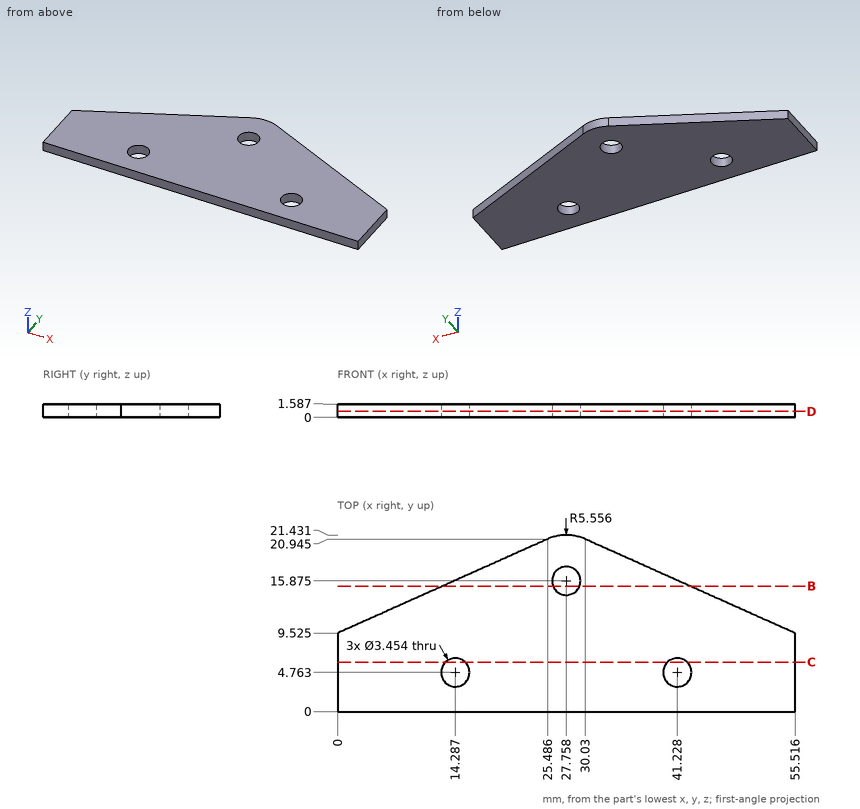
Answer from the drawing. Dimensions are ordinates in mm from the lowest x, y and z of the part. Give positions to 0.01 mm unless a question says otherwise; leave off trailing zeros. Write each loop counter-clockwise with the first axis right and the second up, starting at its lowest first coordinate (ties: lowest second). Pieces come first, ordered by that corner, then holes. Notation, with made-up numbers: M 35,-27.5 L 84,-27.5 A25 cw 84,7.5 Z; hole C 37,47.5 d2. An arc over 180 degrees is marked long. Answer as CSV lines item,"result".
Q1. A cutting plane is placed at C-C on y = 6. Write down the section's boundary in (x, z) (1 decimal).
A:
outline,"M 0,0 L 13.1,0 L 13.1,1.6 L 0,1.6 Z; M 15.5,0 L 40,0 L 40,1.6 L 15.5,1.6 Z; M 42.4,0 L 55.5,0 L 55.5,1.6 L 42.4,1.6 Z"
Q2. A cutting plane is placed at B-B on y = 15.25. Write down the section's boundary in (x, z) (1 decimal).
A:
outline,"M 12.8,0 L 26.1,0 L 26.1,1.6 L 12.8,1.6 Z; M 29.4,0 L 42.7,0 L 42.7,1.6 L 29.4,1.6 Z"
Q3. A cutting plane is placed at D-D on z = 0.7. Write down the section's boundary in (x, y) (1 decimal).
A:
outline,"M 0,0 L 55.5,0 L 55.5,9.5 L 30,20.9 A5.6 ccw 25.5,20.9 L 0,9.5 Z; hole C 14.3,4.8 d3.5; hole C 27.8,15.9 d3.5; hole C 41.2,4.8 d3.5"
Q4. Find the intervals of material crossed by probe 1 along X at (y, z) = (4, 1.4) (1 decimal); probe 2 along Y at (x, z) = (15, 0.35) (1 decimal); probe 3 along Y at (x, z) = (27.5, 1.5) (1 decimal), in increasing order. Write a range as [from, to].
A:
probe 1,"x = [0, 12.7], [15.8, 39.7], [42.8, 55.5]"
probe 2,"y = [0, 3.2], [6.3, 16.2]"
probe 3,"y = [0, 14.2], [17.6, 21.4]"
Q5. Given P1, Ø3, axis at x = 41.23, y = 4.76, coming from the +Z side, flat-ended and moving along its own axis, determine where the tip first touches the part or whether it passes through.
A:
P1,"passes through"
